Print and shaded views of the part. All mm, measured from the part's lowest x, y and z. A direction names the side the tool comes from. Give positions to 0.01 mm unless a question says otherwise; leave off trailing zeros. Loops run counter-clockwise (first coordinate to the right, second up) from the corner with the lowest first, then second, coordinate; pieces in that order, holes last.
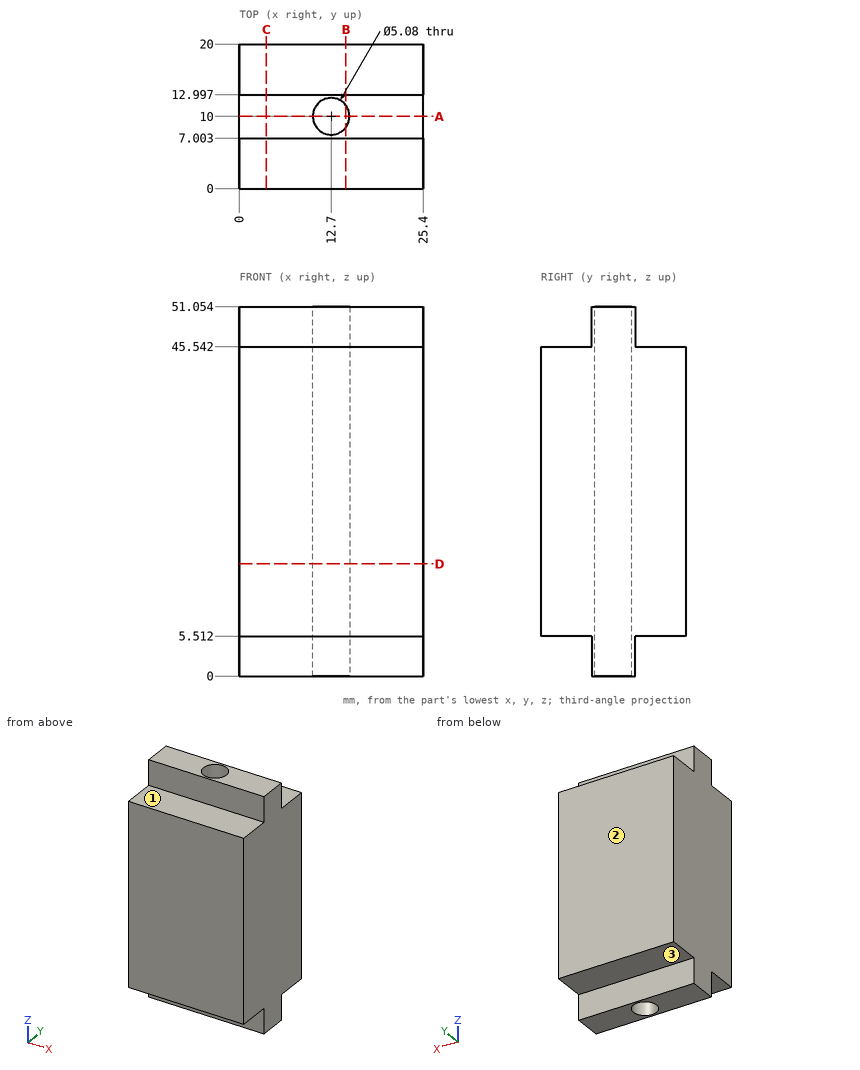
1. Saw through at A-A, the plane y = 10. List the corners of the cut face in (x, z).
Responses:
outline: (0, 0) - (10.16, 0) - (10.16, 51.05) - (0, 51.05) - close; (15.24, 0) - (25.4, 0) - (25.4, 51.05) - (15.24, 51.05) - close
2. Saw through at C-C, the plane x = 3.75. List the corners of the cut face in (y, z), and give its area (3 significant figures).
Responses:
outline: (0, 5.51) - (7, 5.51) - (7, 0) - (13, 0) - (13, 5.51) - (20, 5.51) - (20, 45.54) - (13, 45.54) - (13, 51.05) - (7, 51.05) - (7, 45.54) - (0, 45.54) - close
area: 867 mm2
3. Drop flat-ended pins along their axis: pin 1 (6 mm diameter, centred on x = 18.5, z = 49, fed in from -Y); pin 2 (5 mm diameter, centred on x = 3, z = 35, fed in from -Y); pin 3 (4.5 mm diameter, centred on x = 8, z = 2, fed in from +Y); pin 4 (7.5 mm diameter, centred on x = 14.5, y = 3, fed in from -Z). Give the stop position or say it passes through.
Responses:
pin 1: stops at y = 7
pin 2: stops at y = 0
pin 3: stops at y = 13
pin 4: stops at z = 5.51
4. Probe line 1 along Y through (x, z) = (12.7, 36); line 2 along Z through (x, y) = (17.5, 16); line 3 along X through (y, z) = (9.75, 5). List the from-to ranges inside material, lowest first.
Responses:
line 1: y = 0 to 7.46, 12.54 to 20
line 2: z = 5.51 to 45.54
line 3: x = 0 to 10.17, 15.23 to 25.4
5. Tool access for the marked faces 1, 2 and 3: list every direction of +Z, -Z, +X, -X, +Y, -Y with a clear straight run to the whole face (end or side of a thin tool).
Responses:
face 1: +Z, +X, -X, -Y
face 2: +Z, -Z, +X, -X, +Y
face 3: -Z, +X, -X, +Y
6. Saw through at D-D, the plane z = 15.5. List the corners of the cut face in (x, y), and give its area (3 significant figures).
Responses:
outline: (0, 0) - (25.4, 0) - (25.4, 20) - (0, 20) - close; hole circle Ø5.08 at (12.7, 10)
area: 488 mm2
7. Saw through at B-B, the plane x = 14.75. List the corners of the cut face in (y, z).
Responses:
outline: (0, 5.51) - (7, 5.51) - (7, 0) - (8.5, 0) - (8.5, 51.05) - (7, 51.05) - (7, 45.54) - (0, 45.54) - close; (11.5, 0) - (13, 0) - (13, 5.51) - (20, 5.51) - (20, 45.54) - (13, 45.54) - (13, 51.05) - (11.5, 51.05) - close
